Autodesk Fusion 360 part; units mm, degrees
sketch "Sketch1" plane through (0, 0, 0) normal (0, 0, 1) x (1, 0, 0)
  line L0 (6, 0) -> (674, 0)
  line L1 (680, 6) -> (680, 144)
  line L2 (674, 150) -> (6, 150)
  line L3 (0, 144) -> (0, 6)
  arc A0 (6, 150) -> (0, 144) centre (6, 144) ccw
  arc A1 (680, 144) -> (674, 150) centre (674, 144) ccw
  arc A2 (674, 0) -> (680, 6) centre (674, 6) ccw
  arc A3 (0, 6) -> (6, 0) centre (6, 6) ccw
  point P0 (680, 0)
  point P1 (0, 150)
  dimension "d44" = 680
  dimension "d45" = 150
  dimension "d46" = 6
extrude "Extrude4" add sketch "Sketch1" along normal blind 14
sketch "pf" plane through (0, 0, 14) normal (0, 0, 1) x (1, 0, 0)
  arc A0 (66, 58) -> (90, 58) centre (78, 58) ccw
  arc A1 (0, 144) -> (6, 150) centre (6, 144) cw
  arc A2 (680, 6) -> (674, 0) centre (674, 6) cw
  line L0 (636, 45) -> (636, 130)
  line L1 (6, 150) -> (46, 150)
  line L2 (656, 150) -> (674, 150)
  line L3 (0, 6) -> (0, 144)
  arc A3 (612, 45) -> (636, 45) centre (624, 45) ccw
  arc A4 (636, 130) -> (656, 150) centre (656, 130) cw
  line L4 (680, 144) -> (680, 6)
  arc A5 (90, 130) -> (110, 150) centre (110, 130) cw
  line L5 (612, 130) -> (612, 45)
  line L6 (110, 150) -> (592, 150)
  arc A6 (592, 150) -> (612, 130) centre (592, 130) cw
  arc A7 (46, 150) -> (66, 130) centre (46, 130) cw
  arc A8 (6, 0) -> (0, 6) centre (6, 6) cw
  arc A9 (674, 150) -> (680, 144) centre (674, 144) cw
  line L7 (674, 0) -> (6, 0)
  line L8 (66, 130) -> (66, 58)
  line L9 (90, 58) -> (90, 130)
extrude "Extrude5" add sketch "pf" along normal blind 4
Geometry: final body of the model. Coordinates: model frame, mm. A direction names the side the tool comes from. Give positions to 0.01 mm unless a question says otherwise; leave off trailing zeros. Write each loop counter-clockwise with the first axis right and the second up, starting at its lowest first coordinate (ties: lowest second). Pieces come first, ordered by that corner, then holes.
(1) Cut plane C-C, the plane x = 624. Return loops of the section in (y, z).
(2) Access query for faces 4 (the cylindrical face through (605.986, 144.297, 15.972)), 5 (the flat face through (335, 76, 18)). Directions: +Z, -Z, +X, -X, +Y, -Y. A direction counts if a zero-diameter tool reaches every point of the face in a straight line with its end or side. Return the directions, or none.
(3) Cut plane A-A, the plane y = 87.5. Return loops of the section in (x, z).
(4) Ray query, line 1 (Z direction, x = 628, y = 111). Return the intervals inside material, ascending.
(5) Cut plane B-B, the plane x = 78. Return loops of the section in (y, z), then the cut area to 3 significant figures.
(6) First-contact query: P1, Ø2, axis at x = 360.5, y = 22.5, coming from the -Z side. Flat tip, straight axial feed; report the tip coordinate or a pass-through.
(7) Mould query, pull axis X, two halves, no side actions, for faces 1 (the flat face through (680, 74, 9)), 2 (the flat face through (78, 106, 14)), 3 (the flat face through (335, 76, 0)). Classes: released by +X, released by -X, zero draft, split by the parting line, or undercut.
Values follow:
1. outline: (0, 0) - (150, 0) - (150, 14) - (33, 14) - (33, 18) - (0, 18) - close
2. face 4: +Z, +Y
2. face 5: +Z, +X, -X, +Y, -Y
3. outline: (0, 0) - (680, 0) - (680, 18) - (636, 18) - (636, 14) - (612, 14) - (612, 18) - (90, 18) - (90, 14) - (66, 14) - (66, 18) - (0, 18) - close
4. line 1: z = 0 to 14
5. outline: (0, 0) - (150, 0) - (150, 14) - (46, 14) - (46, 18) - (0, 18) - close
5. area: 2,280 mm2
6. P1: stops at z = 0
7. face 1: released by +X
7. face 2: undercut
7. face 3: zero draft
